Check sheet for the drawn part. Datum: minimum x, y, z corner. Units: mm. Coordinates: 2 decimals unless noted, no trailing zeros. Order: outer loops, then holes, each group sorted by start corner. A loop starts at its lowest first (then second) coordinate and runs counter-clockwise, first axis right, second up. Notation, with made-up numbers: M -25.75,25 L -0.75,25 A35 ccw -0.75,61 Z; hole C 69.5,32 d10. An arc over 180 degrees is marked long. Return JSON: item names as keys, results as strings. Group by question number.
Q1. Section check C-C, the plane x = 2.45. Enter the section's corners in (y, z).
Q2. Section check A-A, the plane y = 6.35. Enter the section's corners in (x, z) (1 decimal).
Q3. Section check B-B, the plane z = 31.75. Enter the section's corners in (x, y) (1 decimal).
Q4. Go/stop test with a flat-tipped pin: pin 1 Ø8 at (y, z) = (30, 4) entering from -X. Record where the tip stops, or that it passes through.
Q5. Thickness scan on probe 1 along Y at (x, z) = (2.1, 31.75); probe 2 along Z at (x, y) = (2.65, 7.5); probe 3 along Y at (x, z) = (0.65, 20.5). Record the ranges inside material, lowest first.
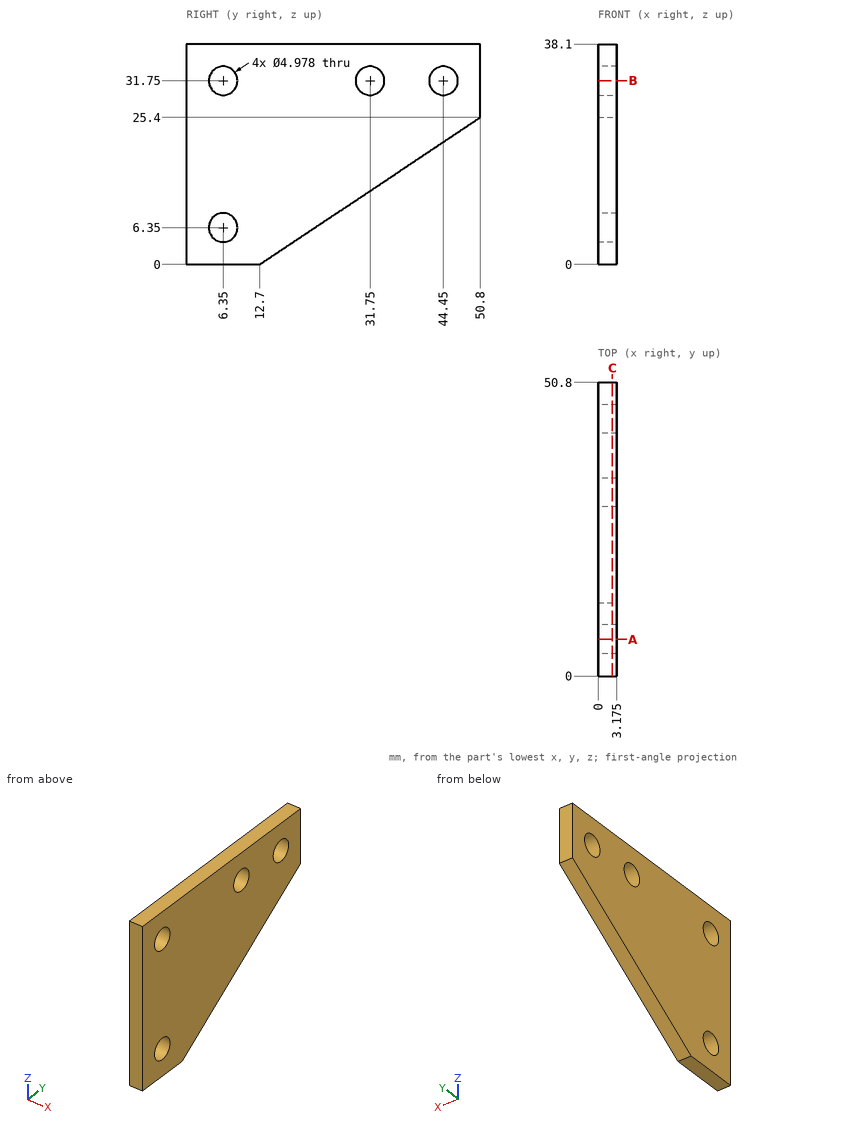
Numbers:
{
 "1": {"outline": "M 0,0 L 12.7,0 L 50.8,25.4 L 50.8,38.1 L 0,38.1 Z; hole C 6.35,6.35 d4.98; hole C 6.35,31.75 d4.98; hole C 31.75,31.75 d4.98; hole C 44.45,31.75 d4.98"},
 "2": {"outline": "M 0,0 L 3.2,0 L 3.2,3.9 L 0,3.9 Z; M 0,8.8 L 3.2,8.8 L 3.2,29.3 L 0,29.3 Z; M 0,34.2 L 3.2,34.2 L 3.2,38.1 L 0,38.1 Z"},
 "3": {"outline": "M 0,0 L 3.2,0 L 3.2,3.9 L 0,3.9 Z; M 0,8.8 L 3.2,8.8 L 3.2,29.3 L 0,29.3 Z; M 0,34.2 L 3.2,34.2 L 3.2,42 L 0,42 Z; M 0,46.9 L 3.2,46.9 L 3.2,50.8 L 0,50.8 Z"},
 "4": {"pin 1": "passes through"},
 "5": {"probe 1": "y = 0 to 3.86, 8.84 to 29.26, 34.24 to 41.96, 46.94 to 50.8", "probe 2": "z = 0 to 4.14, 8.56 to 29.54, 33.96 to 38.1", "probe 3": "y = 0 to 43.45"}
}
